Autodesk Inventor part; units mm, degrees
ref_plane "YZ Plane" through (0, 0, 0) normal (1, 0, 0) x (0, 1, 0)
ref_plane "XZ Plane" through (0, 0, 0) normal (0, 1, 0) x (-1, 0, 0)
ref_plane "XY Plane" through (0, 0, 0) normal (0, 0, 1) x (1, 0, 0)
sketch "Sketch2" plane through (0, 0, 0) normal (0, 1, 0) x (-1, 0, 0)
  line L0 (-15, 15) -> (15, 15)
  line L1 (15, 15) -> (15, -15)
  line L2 (15, -15) -> (-15, -15)
  line L3 (-15, -15) -> (-15, 15)
  line L4 (-15, 15) -> (15, -15) construction
  line L5 (15, 15) -> (-15, -15) construction
  line L6 (15, 6) -> (27, 6)
  line L7 (27, 6) -> (27, -6)
  line L8 (27, -6) -> (15, -6)
  line L9 (15, -6) -> (15, 6)
  line L10 (0, 15) -> (0, -15)
  line L11 (-15, 6) -> (-27, 6)
  line L12 (-27, 6) -> (-27, -6)
  line L13 (-27, -6) -> (-15, -6)
  line L14 (-15, -6) -> (-15, 6)
  circle A0 centre (21, 0) radius 1.6
  circle A1 centre (-21, 0) radius 1.6
  point P0 (0, 0)
  point P1 (15, 0)
  point P2 (-15, 0)
  point P3 (21, 6)
  point P4 (0, 0)
  dimension "d2" = 30
  dimension "d16" = 12
  dimension "d17" = 3.2
extrude "Extrusion1" add sketch "Sketch2" along normal blind 14
sketch "Sketch3" plane through (0, 14, 0) normal (0, 1, 0) x (1, 0, 0)
  line L0 (-3, -12) -> (3, -12)
  line L1 (3, -12) -> (3, -8.8)
  line L2 (3, -8.8) -> (-3, -8.8)
  line L3 (-3, -8.8) -> (-3, -12)
  line L4 (-3, -12) -> (3, -8.8) construction
  line L5 (3, -12) -> (-3, -8.8) construction
  line L6 (-15, 15) -> (-15, -15)
  line L7 (-15, 0) -> (15, 0)
  line L8 (15, -15) -> (15, 15)
  line L9 (-12, -3) -> (-8.8, -3)
  line L10 (-8.8, -3) -> (-8.8, 3)
  line L11 (-8.8, 3) -> (-12, 3)
  line L12 (-12, 3) -> (-12, -3)
  line L13 (-12, -3) -> (-8.8, 3) construction
  line L14 (-8.8, -3) -> (-12, 3) construction
  line L15 (-15, -15) -> (15, -15)
  line L16 (0, -15) -> (0, 15)
  line L17 (15, 15) -> (-15, 15)
  line L18 (-3, 12) -> (3, 12)
  line L19 (3, 12) -> (3, 8.8)
  line L20 (3, 8.8) -> (-3, 8.8)
  line L21 (-3, 8.8) -> (-3, 12)
  line L22 (12, -3) -> (8.8, -3)
  line L23 (8.8, -3) -> (8.8, 3)
  line L24 (8.8, 3) -> (12, 3)
  line L25 (12, 3) -> (12, -3)
  line L26 (12, -3) -> (8.8, 3) construction
  line L27 (8.8, -3) -> (12, 3) construction
  point P0 (0, 0)
  point P1 (0, -10.4)
  point P2 (-10.4, 0)
  point P3 (0, 0)
  point P4 (10.4, 0)
  dimension "d10" = 3
  dimension "d11" = 3
  dimension "d12" = 6
  dimension "d13" = 3.2
extrude "Extrusion2" cut sketch "Sketch3" against normal through all contours L3 L2 L16 L0 | L16 L2 L1 L0 | L10 L9 L12 L7 | L7 L12 L11 L10 | L23 L24 L25 L7 | L7 L25 L22 L23 | L20 L21 L18 L16 | L16 L18 L19 L20
sketch "Sketch4" plane through (0, 14, 0) normal (0, 1, 0) x (1, 0, 0)
  circle A0 centre (-21, 0) radius 3
  circle A1 centre (-21, 0) radius 1.6
  line L0 (-15, -15) -> (15, -15)
  line L1 (0, -15) -> (0, 15)
  line L2 (15, 15) -> (-15, 15)
  circle A2 centre (21, 0) radius 3
  point P0 (0, 0)
  dimension "d18" = 6
extrude "Extrusion3" cut sketch "Sketch4" against normal blind 4 contours A0 | A1 | A2
fillet "Fillet1" radius 5 4 edges at (15, 7, -6) (15, 7, 6) (-15, 7, 6) (-15, 7, -6)
sketch "Sketch5" plane through (0, 14, 0) normal (0, 1, 0) x (1, 0, 0)
  line L0 (5, 5) -> (-5, 5)
  line L1 (-5, 5) -> (-5, -5)
  line L2 (-5, -5) -> (5, -5)
  line L3 (5, -5) -> (5, 5)
  line L4 (5, 5) -> (-5, -5) construction
  line L5 (-5, 5) -> (5, -5) construction
  point P0 (0, 0)
  dimension "d22" = 10
extrude "Extrusion4" cut sketch "Sketch5" against normal through all
equation "\"d11\" = d10"
properties part number "Lower Path Fixation"
Verification items for the finished model (mm, model axes). A direction names the side the tool comes from. Coordinates: 2 decimals unless noted, no trailing zeros. Order: outer loops, then holes, each group sorted by start corner. A loop starts at its lowest first (then second) coordinate and runs counter-clockwise, first axis right, second up.
Item 1: Material ranges on L1, parallel to X at y = 11.6, z = 0; L2, parallel to Z at x = -2.5, y = 8; L3, parallel to Z at x = 10.5, y = 3.5, recorded low to high.
Filled in:
L1: x = -27 to -24, -18 to -12, -8.8 to -5, 5 to 8.8, 12 to 18, 24 to 27
L2: z = -15 to -12, -8.8 to -5, 5 to 8.8, 12 to 15
L3: z = -15 to -3, 3 to 15
Item 2: Access from +Z, -Z, +X, -X, +Y, -Y to the whole of each face (thin tool, end or side, straight path). Record for faces 1 (the face through (-23, 7, 6)), 2 (the face through (-15, 7, -13)), 3 (the face through (12, 7, 0)), 4 (the face through (15, 7, -13)), 5 (the face through (-19.7, 10, 1.3)).
Filled in:
face 1: +Z, -X, +Y, -Y
face 2: -Z, -X, +Y, -Y
face 3: +Y, -Y
face 4: -Z, +X, +Y, -Y
face 5: +Y
Item 3: Section check D-D, the plane x = -9.5. Enter the section's corners in (y, z), then the cut area to 3 significant figures.
Filled in:
outline: (0, -15) - (14, -15) - (14, -3) - (0, -3) - close; (0, 3) - (14, 3) - (14, 15) - (0, 15) - close
area: 336 mm2
Item 4: Release check for a two-part mould opening along Z. For faces 6 (the face through (-6, 14, 0)), 7 (the face through (0, 7, -15)), 8 (the face through (18, 12, 0)) record: +Z half, -Z half, draft (parallel to the pull), parting line (faces both ways), or undercut.
Filled in:
face 6: draft
face 7: -Z half
face 8: undercut
Item 5: Section check B-B, the plane z = 0. Give the number of separate pieces and of enclosed holes in the cut face, then the cut area to 3 significant figures.
Filled in:
separate pieces: 6
enclosed holes: 0
area: 414 mm2
Item 6: Depth check by flat-ended pin: pin 1 (4 mm diameter, centred on x = 21, z = 0, fed in from -Y); pin 2 (3 mm diameter, centred on y = 4.5, z = -13.5, fed in from +X); pin 3 (1 mm diameter, centred on y = 7.5, z = 9.5, fed in from -X); pin 4 (7.5 mm diameter, centred on x = 22.5, y = 4.5, fed in from +Z). Enter the tip coordinate at first touch or a pass-through.
Filled in:
pin 1: stops at y = 0
pin 2: stops at x = 15
pin 3: stops at x = -15.42
pin 4: stops at z = 6.16
Item 7: Section check A-A, the plane x = 21. Enter the section's corners in (y, z).
Filled in:
outline: (0, -6) - (14, -6) - (14, -3) - (10, -3) - (10, -1.6) - (0, -1.6) - close; (0, 1.6) - (10, 1.6) - (10, 3) - (14, 3) - (14, 6) - (0, 6) - close
